```python
from build123d import *

# Parameters (mm, degrees)
BOSS_EXTRUDE1_DEPTH     = 2133.6
SKETCH2_W               = 42.970576624
SKETCH2_H               = 44.626294369
BOSS_EXTRUDE2_DEPTH     = 10
CUT_EXTRUDE1_DEPTH      = 2134.6
CUT_EXTRUDE1_DEPTH_BACK = 1


with BuildPart() as part:
    # Sketch1 → Boss-Extrude1 (new body)
    with BuildSketch(Plane(origin=(0, 0, 0), x_dir=(1, 0, 0), z_dir=(0, 1, 0))):
        with BuildLine():
            Line((13.630161568, 10), (23.630161568, 10))
            ThreePointArc((23.630161568, 10), (29.962715696, 8.909575546), (34.999417241, 4.919349386))
            ThreePointArc((34.999417241, 4.919349386), (36.697471107, 1.472711464), (36.970576624, -2.359795976))
            Line((36.970576624, -2.359795976), (33.961097926, -26.870033055))
            ThreePointArc((33.961097926, -26.870033055), (33.301245719, -28.12420581), (31.976005623, -28.626294369))
            Line((31.976005623, -28.626294369), (5.284317513, -28.626294369))
            ThreePointArc((5.284317513, -28.626294369), (3.959077417, -28.12420581), (3.29922521, -26.870033055))
            Line((3.29922521, -26.870033055), (0.298191514, -2.428574989))
            ThreePointArc((0.298191514, -2.428574989), (0.53721959, 1.274672171), (2.110183266, 4.635767116))
            ThreePointArc((2.110183266, 4.635767116), (7.170061398, 8.821409583), (13.630161568, 10))
        make_face()
    extrude(amount=BOSS_EXTRUDE1_DEPTH)

    # Sketch2 → Boss-Extrude2 (add)
    with BuildSketch(Plane(origin=(0, 0, 0), x_dir=(1, 0, 0), z_dir=(0, 1, 0))):
        with Locations((18.485288312, -9.313147185)):
            Rectangle(SKETCH2_W, SKETCH2_H)
    extrude(amount=BOSS_EXTRUDE2_DEPTH)

    # Sketch3 → Cut-Extrude1 (cut, two sides)
    with BuildSketch(Plane(origin=(0, 0, 0), x_dir=(1, 0, 0), z_dir=(0, 1, 0))) as cut_extrude1_sk:
        with BuildLine():
            Line((0.298191514, -2.428574989), (3.29922521, -26.870033055))
            ThreePointArc((3.29922521, -26.870033055), (3.959077417, -28.12420581), (5.284317513, -28.626294369))
            Line((5.284317513, -28.626294369), (31.976005623, -28.626294369))
            ThreePointArc((31.976005623, -28.626294369), (33.301245719, -28.12420581), (33.961097926, -26.870033055))
            Line((33.961097926, -26.870033055), (36.970576624, -2.359795976))
            ThreePointArc((36.970576624, -2.359795976), (36.697471107, 1.472711464), (34.999417241, 4.919349386))
            ThreePointArc((34.999417241, 4.919349386), (29.962715696, 8.909575546), (23.630161568, 10))
            Line((23.630161568, 10), (13.630161568, 10))
            ThreePointArc((13.630161568, 10), (7.170061398, 8.821409583), (2.110183266, 4.635767116))
            ThreePointArc((2.110183266, 4.635767116), (0.53721959, 1.274672171), (0.298191514, -2.428574989))
        make_face()
    extrude(amount=CUT_EXTRUDE1_DEPTH, mode=Mode.SUBTRACT)
    extrude(cut_extrude1_sk.sketch, amount=-CUT_EXTRUDE1_DEPTH_BACK, mode=Mode.SUBTRACT)


solid = part.part
```
Verification items for the finished model (mm, model axes). A direction names the side the tool comes from. Give positions to 0.01 mm unless a question says otherwise; leave off trailing zeros. Order: outer loops, then holes, each group sorted by start corner. A loop starts at its lowest first (then second) coordinate and runs counter-clockwise, first axis right, second up. Notation, with made-up numbers: (-26, 21) - (-4, 21) arc R24 cw to (-4, 45) - close; hole circle Ø3 at (12, 22.5). An arc over 180 degrees is marked (long way). Answer as CSV lines item,"result". Start each with the question number.
Item 1: Material ranges on L1, parallel to Z at x = 14, y = 4.25; L2, parallel to X at y = 6.25, z = 1.5; L3, parallel to X at y = 8.5, z = 20, recorded low to high.
Item 2: Section check A-A, the plane y = 4.75. Record the boundary of the cut face in (x, z).
Item 3: Access from +Z, -Z, +X, -X, +Y, -Y to the whole of each face (thin tool, end or side, straight path). Record for faces 4 (the face through (1.778, 4.93, 14.478)), 5 (the face through (18, 5, -13)).
Item 4: Section check C-C, the plane z = -2. Record the boundary of the cut face in (x, y), plus the area to 3 significant figures.
Item 5: Section check B-B, the plane x = 21.5. Record the boundary of the cut face in (y, z), plus the area to 3 significant figures.
Item 6: Mould release check, pull along Z, two halves, no side actions. Record for faces 1 (the face through (37, 10, 9)), 2 (the face through (18, 5, 31.626)), 3 (the face through (30.05, 4.93, -8.87)): released by +Z, released by -Z, zero draft, split by the parting line, or undercut.
Filled in:
1,L1,"-13 to -10, 28.63 to 31.63"
1,L2,"-3 to 0.23, 37.04 to 39.97"
1,L3,"-3 to 2.46, 34.8 to 39.97"
2,outline,"(-3, -13) - (39.97, -13) - (39.97, 31.63) - (-3, 31.63) - close; hole (0.3, 2.43) arc R10 ccw to (2.11, -4.64) arc R13 ccw to (13.63, -10) - (23.63, -10) arc R13 ccw to (35, -4.92) arc R10 ccw to (36.97, 2.36) - (33.96, 26.87) arc R2 ccw to (31.98, 28.63) - (5.28, 28.63) arc R2 ccw to (3.3, 26.87) - close"
3,face 4,"+Y, -Y"
3,face 5,"-Z, +X, -X, +Y, -Y"
4,outline,"(-3, 0) - (0.75, 0) - (0.75, 10) - (-3, 10) - close; (36.54, 0) - (39.97, 0) - (39.97, 10) - (36.54, 10) - close"
4,area,"71.8 mm^2"
5,outline,"(0, -13) - (10, -13) - (10, -10) - (0, -10) - close; (0, 28.63) - (10, 28.63) - (10, 31.63) - (0, 31.63) - close"
5,area,"60.0 mm^2"
6,face 1,"zero draft"
6,face 2,"released by +Z"
6,face 3,"undercut"
